from build123d import *

# Parameters (mm, degrees)
EXTRUDE_1_DEPTH          = 10
EXTRUDE_2_DEPTH          = 10
SKETCH_3_R               = 2.25
CUT_EXTRUDE_1_DEPTH      = 5.049845
CUT_EXTRUDE_1_DEPTH_BACK = 4
SKETCH_4_R               = 2.25
CUT_EXTRUDE_2_DEPTH      = 4
FILLET_1_R               = 3
FILLET_2_R               = 1


with BuildPart() as part:
    # Эскиз1 → Бобышка-Вытянуть1 (new body)
    with BuildSketch(Plane(origin=(0, 0, 0), x_dir=(1, 0, 0), z_dir=(0, 1, 0))):
        with BuildLine():
            Line((0, 0), (0, 8))
            ThreePointArc((0, 8), (-7.1, 15.1), (0, 22.2))
            Line((0, 22.2), (0, 37.8))
            ThreePointArc((0, 37.8), (-7.1, 44.9), (0, 52))
            Line((0, 52), (0, 60))
            Line((0, 60), (-3, 60))
            Line((-3, 60), (-3, 54.544169223))
            ThreePointArc((-3, 54.544169223), (-10.1, 44.9), (-3, 35.255830777))
            Line((-3, 35.255830777), (-3, 24.744169223))
            ThreePointArc((-3, 24.744169223), (-10.1, 15.1), (-3, 5.455830777))
            Line((-3, 5.455830777), (-3, 0))
            Line((-3, 0), (0, 0))
        make_face()
    extrude(amount=EXTRUDE_1_DEPTH)

    # Эскиз2 → Бобышка-Вытянуть2 (add)
    with BuildSketch(Plane(origin=(0, 10, 0), x_dir=(1, 0, 0), z_dir=(0, 1, 0))):
        with BuildLine():
            Line((-3, 60), (-8.049844719, 60))
            Line((-8.049844719, 60), (-8.049844719, 51))
            ThreePointArc((-8.049844719, 51), (-5.802159163, 53.167100402), (-3, 54.544169223))
            Line((-3, 54.544169223), (-3, 60))
        make_face()
        with BuildLine():
            Line((-3, 0), (-3, 5.455830777))
            ThreePointArc((-3, 5.455830777), (-5.802159163, 6.832899598), (-8.049844719, 9))
            Line((-8.049844719, 9), (-8.049844719, 0))
            Line((-8.049844719, 0), (-3, 0))
        make_face()
    extrude(amount=-EXTRUDE_2_DEPTH)

    # Эскиз3 → Вырез-Вытянуть1 (cut, two sides)
    with BuildSketch(Plane.ZY.offset(3)) as cut_extrude_1_sk:
        with Locations((-55.75, 5)):
            Circle(SKETCH_3_R)
        with Locations((-4.25, 5)):
            Circle(SKETCH_3_R)
    extrude(amount=CUT_EXTRUDE_1_DEPTH, mode=Mode.SUBTRACT)
    extrude(cut_extrude_1_sk.sketch, amount=-CUT_EXTRUDE_1_DEPTH_BACK, mode=Mode.SUBTRACT)

    # Эскиз4 → Вырез-Вытянуть2 (cut, through all)
    with BuildSketch(Plane.ZY.offset(3)):
        with Locations((-30, 5)):
            Circle(SKETCH_4_R)
    extrude(amount=-CUT_EXTRUDE_2_DEPTH, mode=Mode.SUBTRACT)

    # Скругление1
    fillet_1_edges = [part.edges().sort_by_distance(p)[0] for p in [
        (-3, 5, -24.744169223),
        (-3, 5, -35.255830777),
        (-8.049844719, 5, -51),
        (-8.049844719, 5, -9),
    ]]
    fillet(fillet_1_edges, radius=FILLET_1_R)

    # Скругление2
    fillet_2_edges = [part.edges().sort_by_distance(p)[0] for p in [
        (-8.049844719, 5, -60),
        (-8.049844719, 5, 0),
    ]]
    fillet(fillet_2_edges, radius=FILLET_2_R)


solid = part.part
Input: part model. Units: mm. Frame: model coordinates. A direction names the side the tool comes from. Round coordinates to 2 decimals unless told otherwise and drop trailing zeros. Order: outer loops, then holes, each group sorted by start corner. A loop starts at its lowest first (then second) coordinate and runs counter-clockwise, first axis right, second up. Notation, with made-up numbers: (17, -13) - (72, -13) arc R21 ccw to (72, 17) - close; hole circle Ø2 at (-28, 83.25). An arc over 180 degrees is marked (long way). Answer as a JSON object with one key per item and string values. Group by question number.
(1) Cut plane D-D (x = -9.25). Return loops of the section in (y, z).
(2) Cut plane A-A (y = 5). Count the separate pieces of the cut face and the enclosed holes in it, then the cut area to 3 significant figures.
(3) Cut plane B-B (z = -30). Return loops of the section in (x, y).
(4) Material intervals for probe 1 along Y at (x, z) = (-1.7, -55.75); probe 2 along Z at (x, y) = (-4.5, 6.5); probe 3 along Z at (x, y) = (-2.75, 8), sorted ascending. Write a range as from..to.
(5) Draft query along Z for faces 4 (the face through (-7.765, 4.93, -59.699)), 5 (the face through (0, 3, -28)), 6 (the face through (-9.78, 4.93, -42.38)), 7 (the face through (-1.521, 5.676, -27.854)). Return one class per face: released by +Z, released by -Z, zero draft, split by the parting line, or undercut.
(6) Pin query (flat end, axial travel): P1, Ø1.5, axis at x = -8, y = 1.5, coming from the +Z side; P2, Ø2.5, axis at y = 5, z = -4.25, coming from the +X side; P3, Ø5.5, axis at y = 5, z = -3, coming from the -X side. Return the tip coordinate at first contact, or that it passes through.
(7) Reachability of faces 1 (the face through (-8.05, 7.3, -54.7)), 2 (the face through (-2, 10, -30)), 3 (the face through (-3.43, 5.07, -25.2)) from +Z, -Z, +X, -X, +Y, -Y: full face, straight path, thin tool, end or side. Return the list, or none.
(8) Cut plane C-C (x = -3.75). Return loops of the section in (y, z).
Here are the results:
{
 "1": {"outline": "(0, -48.96) - (10, -48.96) - (10, -40.84) - (0, -40.84) - close; (0, -19.16) - (10, -19.16) - (10, -11.04) - (0, -11.04) - close"},
 "2": {"separate pieces": "4", "enclosed holes": "0", "area": "207 mm^2"},
 "3": {"outline": "(-3, 0) - (0, 0) - (0, 2.75) - (-3, 2.75) - close; (-3, 7.25) - (0, 7.25) - (0, 10) - (-3, 10) - close"},
 "4": {"probe 1": "y = 0..2.75, 7.25..10", "probe 2": "z = -60..-57.43, -54.07..-50.39, -39.41..-35.85, -24.15..-20.59, -9.61..-5.93, -2.57..0", "probe 3": "z = -60..-51.45, -38.35..-21.65, -8.55..0"},
 "5": {"face 4": "released by -Z", "face 5": "zero draft", "face 6": "undercut", "face 7": "undercut"},
 "6": {"P1": "stops at z = -0.02", "P2": "passes through", "P3": "stops at x = -8.05"},
 "7": {"face 1": "-Z, -X, +Y, -Y", "face 2": "+Z, -Z, +X, -X, +Y", "face 3": "-X, +Y, -Y"},
 "8": {"outline": "(0, -60) - (10, -60) - (10, -50.93) - (0, -50.93) - close; (0, -38.87) - (10, -38.87) - (10, -35.24) - (0, -35.24) - close; (0, -24.76) - (10, -24.76) - (10, -21.13) - (0, -21.13) - close; (0, -9.07) - (10, -9.07) - (10, 0) - (0, 0) - close; hole circle Ø4.5 at (5, -55.75); hole circle Ø4.5 at (5, -4.25)"}
}
